Autodesk Inventor part; units mm, degrees
ref_plane "YZ Plane" through (0, 0, 0) normal (1, 0, 0) x (0, 1, 0)
ref_plane "XZ Plane" through (0, 0, 0) normal (0, 1, 0) x (-1, 0, 0)
ref_plane "XY Plane" through (0, 0, 0) normal (0, 0, 1) x (1, 0, 0)
ref_plane "Work Plane1" through (149.76, -42.5858, 44.0081) normal (0, 1, 0) x (-1, 0, 0)
sketch "Sketch1" plane through (149.76, -42.5858, 44.0081) normal (0, 1, 0) x (-1, 0, 0)
  line L0 (106, 4) -> (260, 4)
  line L1 (106, 0) -> (260, 0) construction
  line L2 (106, 0.5) -> (260, 0.5)
  line L3 (106, 6) -> (260, 6)
  line L4 (106, -1.5) -> (260, -1.5)
  line L5 (174.2008, 6) -> (174.2008, 4)
  line L6 (132.2008, -1.5) -> (132.2008, 0.5)
  line L7 (174.2008, 4) -> (174.2008, 0.5)
  line L8 (174.2008, 0.5) -> (174.2008, -1.5)
  line L9 (132.2008, 4) -> (132.2008, 6)
  line L10 (132.2008, 0.5) -> (132.2008, 4)
  point P0 (149.76, -44.0081)
  dimension "d0" = 0.5
  dimension "d1" = 2
  dimension "d2" = 2
  dimension "d3" = 42
extrude "Extrusion1" add sketch "Sketch1" against normal blind 20 contours L9 L3 L5 L0 | L2 L8 L4 L6
sketch "Sketch2" plane through (149.76, -42.5858, 44.0081) normal (0, 1, 0) x (1, 0, 0)
  line L0 (-132.2008, 1.5) -> (-174.2008, 1.5)
  line L1 (-174.2008, 1.5) -> (-174.2008, -0.5)
  line L2 (-174.2008, -4) -> (-174.2008, -0.5)
  line L3 (-174.2008, -4) -> (-174.2008, -6)
  line L4 (-174.2008, -6) -> (-132.2008, -6)
  line L5 (-132.2008, -6) -> (-132.2008, -4)
  line L6 (-132.2008, -0.5) -> (-132.2008, -4)
  line L7 (-132.2008, -0.5) -> (-132.2008, 1.5)
  point P0 (-149.76, 44.0081)
extrude "Extrusion2" add sketch "Sketch2" along normal blind 2
sketch "Sketch3" plane through (17.5592, -62.5858, 42.5081) normal (0, 0, -1) x (-1, 0, 0)
  line L0 (0, 20) -> (0, 0)
  line L1 (0, 2) -> (42, 2) construction
  line L2 (42, 20) -> (42, 0)
  line L3 (42, 0) -> (0, 0)
  line L4 (28.1005, 0) -> (42, 13.8995)
  point P0 (17.5592, 62.5858)
  point P1 (40, 2)
  point P2 (14, 2)
  dimension "d8" = 2
  dimension "d12" = 7
  dimension "d23" = 45
  dimension "d24" = 2
  dimension "d25" = 26
hole "Hole1" at (3.5592, -60.5858, 42.5081) at (-22.4408, -60.5858, 42.5081) direction (0, 0, 1) diameter 2.4 end through all counterbore diameter 6 counterbore depth 6.35
sketch "Sketch4" plane through (17.5592, -40.5858, 42.5081) normal (0, 0, -1) x (-1, 0, 0)
  line L0 (0, -2) -> (0, -22)
  line L1 (42, -22) -> (0, -22)
  line L2 (28.1005, -22) -> (42, -8.1005)
  point P0 (17.5592, 40.5858)
extrude "Extrusion3" cut sketch "Sketch3" against normal up to surface (2 mm away)
properties part number "display_holder"
Geometry: final body of the model. Coordinates: model frame, mm. A direction names the side the tool comes from. Coordinates: 2 decimals unless noted, no trailing zeros. Order: outer loops, then holes, each group sorted by start corner. A loop starts at its lowest first (then second) coordinate and runs counter-clockwise, first axis right, second up.
Item 1: Section query A-A (y = -45.5). Output: boundary loops of the cut face in (x, z).
Answer:
outline: (-24.44, 42.51) - (17.56, 42.51) - (17.56, 44.51) - (-24.44, 44.51) - close; (-24.44, 48.01) - (17.56, 48.01) - (17.56, 50.01) - (-24.44, 50.01) - close
Item 2: Section query C-C (z = 43.5). Output: boundary loops of the cut face in (x, y), then the cut area to 3 significant figures.
Answer:
outline: (-24.44, -48.69) - (-10.54, -62.59) - (1.32, -62.59) arc R3 cw (long way) to (5.8, -62.59) - (17.56, -62.59) - (17.56, -40.59) - (-24.44, -40.59) - close
area: 802 mm2
Item 3: Contact query for flat-ended pins moving along their axis: P1, Ø5, axis at x = 3.56, y = -60.59, coming from the +Z side; P2, Ø2, axis at x = -22.44, y = -60.59, coming from the -Z side; P3, Ø2.5, axis at x = -22.5, y = -61, coming from the -Z side; P4, Ø1.8, axis at x = -2, z = 45.5, coming from the -Y side. Output: stop coordinate, or through.
Answer:
P1: stops at z = 50.01
P2: passes through
P3: stops at z = 48.86
P4: stops at y = -42.59
Item 4: Access query for faces 4 (the face through (12, -62.586, 44)), 5 (the face through (-17.394, -55.733, 43.494)), 6 (the face through (4, -59, 48.858)), 7 (the face through (-3, -52, 48.008)). Directions: +Z, -Z, +X, -X, +Y, -Y. A direction counts if a zero-diameter tool reaches every point of the face in a straight line with its end or side. Return the directions, or none.
Answer:
face 4: +Z, -Z, +X, -X, -Y
face 5: -Z, -X, -Y
face 6: -Z
face 7: +X, -X, -Y
Item 5: Draft query along Y for faces 1 (the face through (17.559, -52, 49)), 2 (the face through (-20.275, -58.51, 48.439)), 3 (the face through (-3, -62.586, 49)). Return one class per face: released by +Y, released by -Y, zero draft, split by the parting line, or undercut.
Answer:
face 1: zero draft
face 2: undercut
face 3: released by -Y
Item 6: Section query B-B (x = 13). Output: boundary loops of the cut face in (y, z).
Answer:
outline: (-62.59, 42.51) - (-40.59, 42.51) - (-40.59, 50.01) - (-62.59, 50.01) - (-62.59, 48.01) - (-42.59, 48.01) - (-42.59, 44.51) - (-62.59, 44.51) - close
Item 7: Section query D-D (y = -61). Output: boundary loops of the cut face in (x, z).
Answer:
outline: (-24.44, 48.86) - (-23.57, 48.86) - (-23.57, 50.01) - (-24.44, 50.01) - close; (-21.31, 48.86) - (-19.47, 48.86) - (-19.47, 48.01) - (0.59, 48.01) - (0.59, 48.86) - (2.43, 48.86) - (2.43, 50.01) - (-21.31, 50.01) - close; (-12.13, 42.51) - (0.59, 42.51) - (0.59, 44.51) - (-12.13, 44.51) - close; (4.69, 48.86) - (6.53, 48.86) - (6.53, 48.01) - (17.56, 48.01) - (17.56, 50.01) - (4.69, 50.01) - close; (6.53, 42.51) - (17.56, 42.51) - (17.56, 44.51) - (6.53, 44.51) - close
Item 8: Material intervals for line 1 along Z through (x, y) = (12.5, -54.5); line 2 along Y through (x, z) = (13.5, 44.75); line 3 along X through (y, z) = (-61.25, 48.25), sorted ascending.
Answer:
line 1: z = 42.51 to 44.51, 48.01 to 50.01
line 2: y = -42.59 to -40.59
line 3: x = -19.52 to 0.63, 6.48 to 17.56
